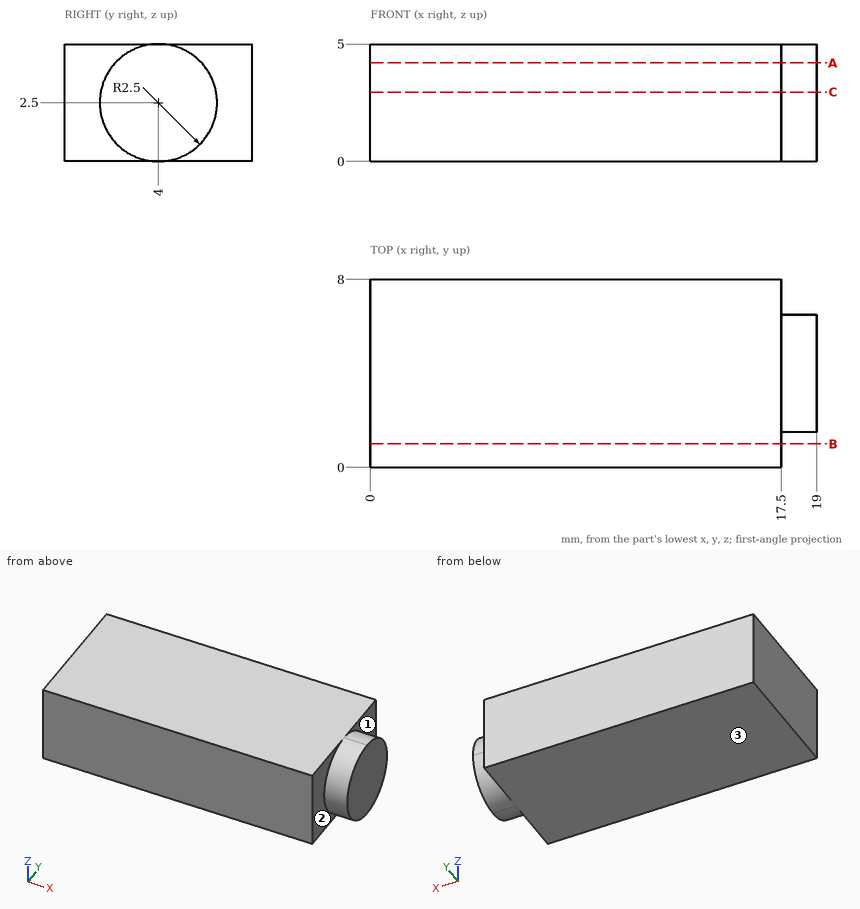
Input: dimensioned drawing with shaded views. Units: mm. Origin: part minimum x, y, z. A direction names the side the tool comes from. Round coordinates to 2 decimals unless told otherwise and drop trailing zeros. Order: outer loops, then holes, each group sorted by start corner. A loop starts at its lowest first (then second) coordinate and runs counter-clockwise, first axis right, second up.
1. Cut plane B-B, the plane y = 1. Output: boundary loops of the cut face in (x, z), then the cut area to 3 significant figures.
The answers:
outline: (0, 0) - (17.5, 0) - (17.5, 5) - (0, 5) - close
area: 87.5 mm2
2. Material intervals for line 1 (X direction, y = 7, z = 4.15); line 2 (Y direction, x = 18.25, z = 3.55), sorted ascending.
The answers:
line 1: x = 0 to 17.5
line 2: y = 1.73 to 6.27
3. Set-up query: the marked faces 1, 2 and 3. Return all of +Z, -Z, +X, -X, +Y, -Y with unobstructed straight access to the full face (end or side cutting, diameter ignored); none if empty.
The answers:
face 1: +X, +Y
face 2: +X, -Y
face 3: -Z, +X, -X, +Y, -Y
4. Cut plane A-A, the plane z = 4.2. Output: boundary loops of the cut face in (x, y), then the cut area to 3 significant figures.
The answers:
outline: (0, 0) - (17.5, 0) - (17.5, 2.17) - (19, 2.17) - (19, 5.83) - (17.5, 5.83) - (17.5, 8) - (0, 8) - close
area: 145 mm2
5. Cut plane C-C, the plane z = 2.95. Output: boundary loops of the cut face in (x, y), then the cut area to 3 significant figures.
The answers:
outline: (0, 0) - (17.5, 0) - (17.5, 1.54) - (19, 1.54) - (19, 6.46) - (17.5, 6.46) - (17.5, 8) - (0, 8) - close
area: 147 mm2
